The model under review builds one solid part; all positions refer to its coordinate system, in mm. A direction names the side the tool comes from. Give positions to 0.01 mm unless a question says otherwise; leave off trailing zeros. Order: outer loops, then holes, each group sorted by start corner. A loop starts at its lowest first (then second) coordinate and runs counter-clockwise, first axis right, second up. Notation, with made-up numbers: (-14, 48) - (25, 48) arc R24 ccw to (25, 72) - close; hole circle Ø4 at (12, 14.25). An arc over 180 degrees is marked (long way). Write item = value, one per line. Start each with the question number.
1. Mouldability with a two-part tool opening along Y and no side actions: class faces 3 (the flat face through (20, -20.638, -451)), 4 (the flat face through (0, 0, -914.4)), 5 (the flat face through (20, 17.844, -451)) as pulls with the +Y half, pulls with the -Y half, needs draft (parallel to the pull), parting line crosses it, or undercut.
2. For P1, Ø1, axis at y = 13, z = -606.5, coming from the -X side; P2, Ø1, axis at y = -11.5, z = -341.5, coming from the +X side; P3, Ø10.5, axis at y = -3.5, z = -241, coming from the +X side, all flat-tipped, find the tip position at first contact; note any pin that passes through.
3. We need section B-B, the plane y = 2. Give the boundary of the cut face in (x, z), and give its area (3 significant figures).
4. Machinability: for faces 1 (the flat face through (20, 20.638, -451)), 2 (the flat face through (2.794, 0, -451)), which of the approach directions +Z, -Z, +X, -X, +Y, -Y give a long, thin tool a straight path to every point of the face, cutting with its end or side? Answer none if there is none.
5. We need section A-A, the plane x = -12.5. Give the boundary of the cut face in (y, z), and give its area (3 significant figures).
6. Wall thickness on probe 1 along X at (y, z) = (-15, -629) (3 decimals); probe 2 along Y at (x, z) = (37, -866.5); probe 3 along Y at (x, z) = (35, -400): over which ranges is each line inside the solid? List them lowest first.
from build123d import *

# Parameters (mm, degrees)
BOSS_EXTRUDE1_DEPTH = 914.4


with BuildPart() as part:
    # Sketch1 → Boss-Extrude1 (new body)
    with BuildSketch(Plane.XY):
        with BuildLine():
            Line((-36.22675, 20.6375), (-3.46075, 20.6375))
            ThreePointArc((-3.46075, 20.6375), (-1.013630207, 19.623869793), (0, 17.17675))
            Line((0, 17.17675), (0, -17.17675))
            ThreePointArc((0, -17.17675), (-1.013630207, -19.623869793), (-3.46075, -20.6375))
            Line((-3.46075, -20.6375), (-36.22675, -20.6375))
            ThreePointArc((-36.22675, -20.6375), (-39.796401808, -19.158901808), (-41.275, -15.58925))
            Line((-41.275, -15.58925), (-41.275, -14.57325))
            ThreePointArc((-41.275, -14.57325), (-40.261369793, -12.126130207), (-37.81425, -11.1125))
            Line((-37.81425, -11.1125), (-35.5346, -11.1125))
            ThreePointArc((-35.5346, -11.1125), (-34.1376, -12.5095), (-35.5346, -13.9065))
            Line((-35.5346, -13.9065), (-37.81425, -13.9065))
            ThreePointArc((-37.81425, -13.9065), (-38.285713446, -14.101786554), (-38.481, -14.57325))
            Line((-38.481, -14.57325), (-38.481, -15.58925))
            ThreePointArc((-38.481, -15.58925), (-37.820745461, -17.183245461), (-36.22675, -17.8435))
            Line((-36.22675, -17.8435), (-3.46075, -17.8435))
            ThreePointArc((-3.46075, -17.8435), (-2.989286554, -17.648213446), (-2.794, -17.17675))
            Line((-2.794, -17.17675), (-2.794, 17.17675))
            ThreePointArc((-2.794, 17.17675), (-2.989286554, 17.648213446), (-3.46075, 17.8435))
            Line((-3.46075, 17.8435), (-36.22675, 17.8435))
            ThreePointArc((-36.22675, 17.8435), (-37.820745461, 17.183245461), (-38.481, 15.58925))
            Line((-38.481, 15.58925), (-38.481, 14.57325))
            ThreePointArc((-38.481, 14.57325), (-38.285713446, 14.101786554), (-37.81425, 13.9065))
            Line((-37.81425, 13.9065), (-35.5346, 13.9065))
            ThreePointArc((-35.5346, 13.9065), (-34.1376, 12.5095), (-35.5346, 11.1125))
            Line((-35.5346, 11.1125), (-37.81425, 11.1125))
            ThreePointArc((-37.81425, 11.1125), (-40.261369793, 12.126130207), (-41.275, 14.57325))
            Line((-41.275, 14.57325), (-41.275, 15.58925))
            ThreePointArc((-41.275, 15.58925), (-39.796401808, 19.158901808), (-36.22675, 20.6375))
        make_face()
    extrude(amount=-BOSS_EXTRUDE1_DEPTH)


with BuildPart() as body_2:
    # Mirror1: mirrored copy
    add(part.part.mirror(Plane(origin=(0, 17.17675, -914.4), x_dir=(0, 0, 1), z_dir=(1, 0, 0))))


with BuildPart() as part_1:
    add(part.part)

    # Combine1: union body 2
    add(body_2.part)


solid = part_1.part
Model answer:
q1.face_3 = pulls with the -Y half
q1.face_4 = needs draft
q1.face_5 = undercut
q2.P1 = -41.1
q2.P2 = 40.13
q2.P3 = 2.79
q3.outline = (-2.79, -914.4) - (2.79, -914.4) - (2.79, 0) - (-2.79, 0) - close
q3.area = 5,110 mm2
q4.face_1 = +Z, -Z, +X, -X, +Y
q4.face_2 = +Z, -Z
q5.outline = (-20.64, -914.4) - (-17.84, -914.4) - (-17.84, 0) - (-20.64, 0) - close; (17.84, -914.4) - (20.64, -914.4) - (20.64, 0) - (17.84, 0) - close
q5.area = 5,110 mm2
q6.probe_1 = -41.275 to -38.481, -2.794 to 2.794, 38.481 to 41.275
q6.probe_2 = -20.58 to -17.71, -13.91 to -11.11, 11.11 to 13.91, 17.71 to 20.58
q6.probe_3 = -20.64 to -17.84, -13.8 to -11.22, 11.22 to 13.8, 17.84 to 20.64
